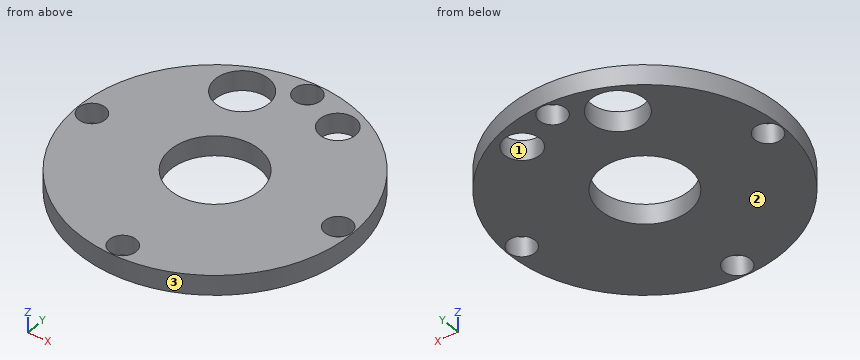
```python
from build123d import *

# Parameters (mm, degrees)
ESQUISSE1_R                  = 30.75
BOSS_EXTRU_1_DEPTH           = 8
ESQUISSE2_R                  = 3
BOSS_EXTRU_2_DEPTH           = 56
ESQUISSE4_R                  = 30.75
BOSS_EXTRU_4_DEPTH           = 4.5
ESQUISSE6_R                  = 3
BOSS_EXTRU_5_DEPTH           = 40
ESQUISSE12_R                 = 4
ENL_V_MAT_EXTRU_1_DEPTH      = 6
ESQUISSE13_R                 = 6
ENL_V_MAT_EXTRU_2_DEPTH      = 10
ESQUISSE15_R                 = 10
ENL_V_MAT_EXTRU_3_DEPTH      = 10
ESQUISSE18_R                 = 30.75
BOSS_EXTRU_10_DEPTH          = 4.5
ESQUISSE19_R                 = 2.05
ENL_V_MAT_EXTRU_4_DEPTH      = 62
ESQUISSE20_R                 = 3.5
ENL_V_MAT_EXTRU_5_DEPTH      = 10
ESQUISSE21_R                 = 3
ENL_V_MAT_EXTRU_6_DEPTH      = 78.376514687
ENL_V_MAT_EXTRU_7_DEPTH      = 122.079003185
ENL_V_MAT_EXTRU_7_DEPTH_BACK = 122.079003185
ESQUISSE22_W                 = 61.5
ESQUISSE22_H                 = 64
ESQUISSE22_H_2               = 4.5


with BuildPart() as part:
    # Esquisse1 → Boss.-Extru.1 (new body)
    with BuildSketch(Plane.XY):
        Circle(ESQUISSE1_R)
    extrude(amount=BOSS_EXTRU_1_DEPTH)

    # Esquisse2 → Boss.-Extru.2 (add)
    with BuildSketch(Plane.XY.offset(8)):
        with Locations((0, 27.5)):
            Circle(ESQUISSE2_R)
        with Locations((27.5, 0)):
            Circle(ESQUISSE2_R)
        with Locations((-27.5, 0)):
            Circle(ESQUISSE2_R)
        with Locations((0, -27.5)):
            Circle(ESQUISSE2_R)
    extrude(amount=BOSS_EXTRU_2_DEPTH)

    # Esquisse4 → Boss.-Extru.4 (add)
    with BuildSketch(Plane.XY.offset(64)):
        Circle(ESQUISSE4_R)
    extrude(amount=BOSS_EXTRU_4_DEPTH)

    # Esquisse6 → Boss.-Extru.5 (add)
    with BuildSketch(Plane.XY.offset(68.5)):
        with Locations((0, -27.5)):
            Circle(ESQUISSE6_R)
        with Locations((-27.5, 0)):
            Circle(ESQUISSE6_R)
        with Locations((0, 27.5)):
            Circle(ESQUISSE6_R)
        with Locations((27.5, 0)):
            Circle(ESQUISSE6_R)
    extrude(amount=BOSS_EXTRU_5_DEPTH)

    # Esquisse12 → Enlèv. mat.-Extru.1 (cut)
    with BuildSketch(Plane.XY.offset(68.5)):
        with Locations((9.98690327, 23.224420757)):
            Circle(ESQUISSE12_R)
    extrude(amount=-ENL_V_MAT_EXTRU_1_DEPTH, mode=Mode.SUBTRACT)

    # Esquisse13 → Enlèv. mat.-Extru.2 (cut)
    with BuildSketch(Plane.XY.offset(68.5)):
        with Locations((-9.931529151, 21.298232995)):
            Circle(ESQUISSE13_R)
    extrude(amount=-ENL_V_MAT_EXTRU_2_DEPTH, mode=Mode.SUBTRACT)

    # Esquisse15 → Enlèv. mat.-Extru.3 (cut)
    with BuildSketch(Plane.XY.offset(68.5)):
        Circle(ESQUISSE15_R)
    extrude(amount=-ENL_V_MAT_EXTRU_3_DEPTH, mode=Mode.SUBTRACT)

    # Esquisse18 → Boss.-Extru.10 (add)
    with BuildSketch(Plane.XY.offset(108.5)):
        Circle(ESQUISSE18_R)
    extrude(amount=BOSS_EXTRU_10_DEPTH)

    # Esquisse19 → Enlèv. mat.-Extru.4 (cut)
    with BuildSketch(Plane.ZY.offset(30.75)):
        with Locations((4, 0.25)):
            Circle(ESQUISSE19_R)
    extrude(amount=-ENL_V_MAT_EXTRU_4_DEPTH, mode=Mode.SUBTRACT)

    # Esquisse20 → Enlèv. mat.-Extru.5 (cut)
    with BuildSketch(Plane.XY.offset(113)):
        with Locations((21.297953152, 14.912987345)):
            Circle(ESQUISSE20_R)
        with Locations((-14.912987345, 21.297953152)):
            Circle(ESQUISSE20_R)
        with Locations((-21.297953152, -14.912987345)):
            Circle(ESQUISSE20_R)
        with Locations((14.912987345, -21.297953152)):
            Circle(ESQUISSE20_R)
    extrude(amount=-ENL_V_MAT_EXTRU_5_DEPTH, mode=Mode.SUBTRACT)

    # Esquisse21 → Enlèv. mat.-Extru.6 (cut, through all)
    with BuildSketch(Plane(origin=(0, 0, 64), x_dir=(-1, 0, 0), z_dir=(0, 0, -1))):
        with Locations((0, 27.5)):
            Circle(ESQUISSE21_R)
        with Locations((-27.5, 0)):
            Circle(ESQUISSE21_R)
        with Locations((0, -27.5)):
            Circle(ESQUISSE21_R)
        with Locations((27.5, 0)):
            Circle(ESQUISSE21_R)
    extrude(amount=-ENL_V_MAT_EXTRU_6_DEPTH, mode=Mode.SUBTRACT)


with BuildPart() as enl_v_mat_extru_6_piece_1:
    # of the separate pieces the step leaves, piece 1, a body of its own (enl_v_mat_extru_6_pieces)
    add(part.part.solids().sort_by_distance((3, -27.5, 8))[0])


with BuildPart() as enl_v_mat_extru_6_piece_2:
    # of the separate pieces the step leaves, piece 2, a body of its own (enl_v_mat_extru_6_pieces)
    add(part.part.solids().sort_by_distance((30.75, 0, 108.5))[0])


with BuildPart() as enl_v_mat_extru_6_piece_3:
    # of the separate pieces the step leaves, piece 3, a body of its own (enl_v_mat_extru_6_pieces)
    add(part.part.solids().sort_by_distance((30.75, 0, 68.5))[0])


with BuildPart() as enl_v_mat_extru_7_tool:
    # Esquisse22 → Enlèv. mat.-Extru.7 (new, two sides: drawn at the far end of the back side and taken through both)
    with BuildSketch(Plane(origin=(0, 0, 0), x_dir=(1, 0, 0), z_dir=(0, 1, 0)).offset(-ENL_V_MAT_EXTRU_7_DEPTH_BACK)):
        with Locations((0, -32)):
            Rectangle(ESQUISSE22_W, ESQUISSE22_H)
        with Locations((0, -110.75)):
            Rectangle(ESQUISSE22_W, ESQUISSE22_H_2)
    extrude(amount=ENL_V_MAT_EXTRU_7_DEPTH + ENL_V_MAT_EXTRU_7_DEPTH_BACK)


with BuildPart() as enl_v_mat_extru_6_piece_1_1:
    add(enl_v_mat_extru_6_piece_1.part)

    # Enlèv. mat.-Extru.7: cut by enl_v_mat_extru_7_tool
    add(enl_v_mat_extru_7_tool.part, mode=Mode.SUBTRACT)


with BuildPart() as enl_v_mat_extru_6_piece_2_1:
    add(enl_v_mat_extru_6_piece_2.part)

    # Enlèv. mat.-Extru.7: cut by enl_v_mat_extru_7_tool
    add(enl_v_mat_extru_7_tool.part, mode=Mode.SUBTRACT)


solid = enl_v_mat_extru_6_piece_3.part
```
The listing builds one solid part. Answer for the finished solid, in the listing's coordinates (mm). Face numbers are marked on the shaded views. Round coordinates to 2 decimals unless told otherwise and drop trailing zeros. Write each loop counter-clockwise with the first axis right and the second up, starting at its lowest first coordinate (ties: lowest second). Pieces come first, ordered by that corner, then holes. Notation, with made-up numbers: (-31, 70) -> (18, 70) arc R36 ccw to (18, 105) -> close; hole circle Ø5 at (-31.5, 23). An arc over 180 degrees is marked (long way). Answer as a JSON object with one key per item and string values. Group by question number.
Q1. Section C-C (y = 17) is taken. Write down the section's boundary in (x, z), plus the area to 3 significant figures.
Q2. Straight lines are drawn through the part: line 1 along Y through (x, z) = (7, 65.6); line 2 along X through (y, z) = (-0.5, 65.3); line 3 along Y through (x, z) = (-7.5, 64.75). For each, find the intervals that lie inside material, in ascending order.
Q3. Section D-D (x = -27.5) is taken. Write down the section's boundary in (y, z).
Q4. This flat-tipped pin is pushed along its axis until it touches: pin 1 Ø7 at (x, y) = (9.99, 23.22) entering from +Z. Where does it stop, or does it pass through?
Q5. Section A-A (x = 0) is taken. Write down the section's boundary in (y, z).
Q6. Determine the mould class of the marked faces 1, 2 and 3 for opening direction X: pulls with the +X half, pulls with the -X half, needs draft (parallel to the pull), parting line crosses it, or undercut.
Check values:
{
 "1": {"outline": "(-25.62, 64) -> (-14.12, 64) -> (-14.12, 68.5) -> (-25.62, 68.5) -> close; (-5.75, 64) -> (25.62, 64) -> (25.62, 68.5) -> (-5.75, 68.5) -> close", "area": "193 mm^2"},
 "2": {"line 1": "-29.94 to -7.14, 7.14 to 20.56, 25.88 to 29.94", "line 2": "-30.75 to -30.46, -24.54 to -9.99, 9.99 to 24.54, 30.46 to 30.75", "line 3": "-29.82 to -6.61, 6.61 to 15.81, 26.78 to 29.82"},
 "3": {"outline": "(-13.76, 64) -> (-3, 64) -> (-3, 68.5) -> (-13.76, 68.5) -> close; (3, 64) -> (13.76, 64) -> (13.76, 68.5) -> (3, 68.5) -> close"},
 "4": {"pin 1": "through"},
 "5": {"outline": "(-30.75, 64) -> (-30.5, 64) -> (-30.5, 68.5) -> (-30.75, 68.5) -> close; (-24.5, 64) -> (-10, 64) -> (-10, 68.5) -> (-24.5, 68.5) -> close; (10, 64) -> (24.5, 64) -> (24.5, 68.5) -> (10, 68.5) -> close; (30.5, 64) -> (30.75, 64) -> (30.75, 68.5) -> (30.5, 68.5) -> close"},
 "6": {"face 1": "undercut", "face 2": "needs draft", "face 3": "parting line crosses it"}
}
